Design review of the part built by this model. Coordinates are the model's own, in mm. Face numbers are marked on the shaded views. A direction names the side the tool comes from. Coordinates: 2 decimals unless noted, no trailing zeros. Write each loop counter-clockwise with the first axis right and the second up, starting at its lowest first coordinate (ties: lowest second). Pieces come first, ordered by that corner, then holes. Notation, with made-up numbers: (59, 17) -> (87, 17) arc R32 cw to (87, 45) -> close; hole circle Ø10 at (-20.75, 80.5). An arc over 180 degrees is marked (long way). One line per question, with ' | ' between items. Start each with the question number.
Q1. Wall thickness on probe 1 along Y at (x, z) = (-32, 45); probe 2 along Z at (x, y) = (2, 35.5): over which ranges is each line inside the solid? List them lowest first.
Q2. Add section B-B on z = 45. State the section outline as (x, y) points, and give its area (3 significant figures).
Q3. For P1, Ø12, axis at y = 11.5, z = 14.5, coming from the -X side; P2, Ø1, axis at x = -31.5, y = -1, coming from the +Z side; P3, Ø1.5, axis at x = -16.5, z = 23.5, coming from the -Y side, all flat-tipped, find the tip position at first contact; note any pin that passes through.
Q4. Add section D-D on z = 24.5. State the section outline as (x, y) points, and give its area (3 significant figures).
Q5. Add section A-A on y = 32. State the section outline as (x, z) points.
Q6. Draft analysis for pull direction X (two halves, no side actions). For the marked faces 1, 2, 3 and 4, state which applies: pulls with the +X half, pulls with the -X half, needs draft (parallel to the pull), parting line crosses it, or undercut.
Q7. For the marked faces 5, 6, 7, 8 and 9, list the 3-axis set-ups (+Z, -Z, +X, -X, +Y, -Y) from which the entire face can be reached by the end or side of a thin tool; tool diameter is ignored.
from build123d import *

# Parameters (mm, degrees)
SKETCH_1_W                = 50
SKETCH_1_H                = 50
SKETCH_1_W_2              = 40.4
SKETCH_1_H_2              = 40.4
EXTRUDE_50_4P8_DEPTH      = 50
SKETCH_2_W                = 80
SKETCH_2_H                = 80
SKETCH_2_W_2              = 40.4
SKETCH_2_H_2              = 40.4
EXTRUDE_379_DEPTH         = 8
EXTRUDE_START             = 42
SKETCH_3_W                = 80
SKETCH_3_H                = 80
SKETCH_3_W_2              = 30
SKETCH_3_H_2              = 30
EXTRUDE_483_DEPTH         = 8
EXTRUDE_START_2           = 50
SKETCH_4_W                = 39.6
SKETCH_4_H                = 39.6
SKETCH_4_W_2              = 30
SKETCH_4_H_2              = 30
EXTRUDE_39P6_DEPTH        = 8
CUT_EXTRUDE_M4_DEPTH      = 82.018516402
CUT_EXTRUDE_M4_DEPTH_BACK = 82.018516402
SKETCH_5_R                = 2.25


with BuildPart() as part:
    # 草图1 → 50方管壁厚4p8 (new body)
    with BuildSketch(Plane.XY):
        Rectangle(SKETCH_1_W, SKETCH_1_H)
        Rectangle(SKETCH_1_W_2, SKETCH_1_H_2, mode=Mode.SUBTRACT)
    extrude(amount=EXTRUDE_50_4P8_DEPTH)

    # 草图2 → Extrude 379 (add)
    with BuildSketch(Plane.XY):
        Rectangle(SKETCH_2_W, SKETCH_2_H)
        Rectangle(SKETCH_2_W_2, SKETCH_2_H_2, mode=Mode.SUBTRACT)
    extrude(amount=EXTRUDE_379_DEPTH)

    # 草图3 → Extrude 483 (add)
    with BuildSketch(Plane.XY.offset(EXTRUDE_START)):
        Rectangle(SKETCH_3_W, SKETCH_3_H)
        Rectangle(SKETCH_3_W_2, SKETCH_3_H_2, mode=Mode.SUBTRACT)
    extrude(amount=EXTRUDE_483_DEPTH)

    # 草图4 → 定位凸台39p6 (add)
    with BuildSketch(Plane.XY.offset(EXTRUDE_START_2)):
        Rectangle(SKETCH_4_W, SKETCH_4_H)
        Rectangle(SKETCH_4_W_2, SKETCH_4_H_2, mode=Mode.SUBTRACT)
    extrude(amount=EXTRUDE_39P6_DEPTH)

    # 草图5 → 四个M4法兰通孔 (cut, two sides: drawn at the far end of the back side and taken through both)
    with BuildSketch(Plane.XY.offset(-CUT_EXTRUDE_M4_DEPTH_BACK)):
        with Locations((-32, -32)):
            Circle(SKETCH_5_R)
        with Locations((-32, 32)):
            Circle(SKETCH_5_R)
        with Locations((32, -32)):
            Circle(SKETCH_5_R)
        with Locations((32, 32)):
            Circle(SKETCH_5_R)
    extrude(amount=CUT_EXTRUDE_M4_DEPTH + CUT_EXTRUDE_M4_DEPTH_BACK, mode=Mode.SUBTRACT)


solid = part.part
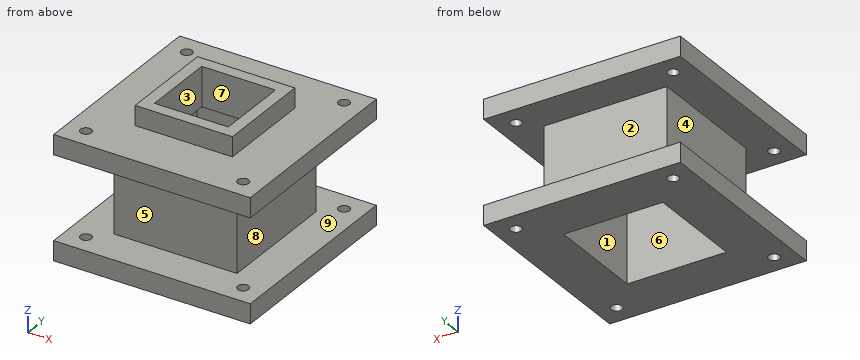
Output values:
1) probe 1: y = -40 to -34.25, -29.75 to 29.75, 34.25 to 40 | probe 2: z = 0 to 8, 42 to 50
2) outline: (-40, -40) -> (40, -40) -> (40, 40) -> (-40, 40) -> close; hole circle Ø4.5 at (-32, -32); hole circle Ø4.5 at (-32, 32); hole (-15, -15) -> (15, -15) -> (15, 15) -> (-15, 15) -> close; hole circle Ø4.5 at (32, -32); hole circle Ø4.5 at (32, 32) | area: 5,440 mm2
3) P1: stops at x = -25 | P2: stops at z = 50 | P3: stops at y = -25
4) outline: (-25, -25) -> (25, -25) -> (25, 25) -> (-25, 25) -> close; hole (-20.2, -20.2) -> (20.2, -20.2) -> (20.2, 20.2) -> (-20.2, 20.2) -> close | area: 868 mm2
5) outline: (-40, 0) -> (-34.25, 0) -> (-34.25, 8) -> (-40, 8) -> close; (-40, 42) -> (-34.25, 42) -> (-34.25, 50) -> (-40, 50) -> close; (-29.75, 0) -> (29.75, 0) -> (29.75, 8) -> (-29.75, 8) -> close; (-29.75, 42) -> (29.75, 42) -> (29.75, 50) -> (-29.75, 50) -> close; (34.25, 0) -> (40, 0) -> (40, 8) -> (34.25, 8) -> close; (34.25, 42) -> (40, 42) -> (40, 50) -> (34.25, 50) -> close
6) face 1: undercut | face 2: needs draft | face 3: undercut | face 4: pulls with the -X half
7) face 5: +X, -X, -Y | face 6: -Z | face 7: +Z, -Z | face 8: +X, +Y, -Y | face 9: none
